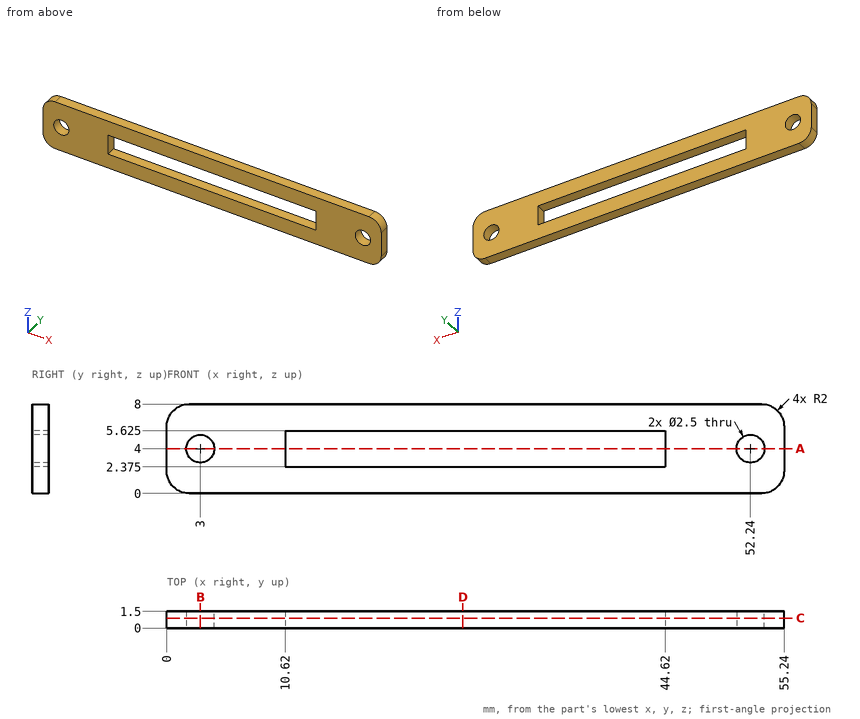
Here's the drawing with two shaded views (mm, measured from the low corner). I have some questions. Round coordinates to 2 decimals unless told otherwise and drop trailing zeros. Loops run counter-clockwise (first coordinate to the right, second up) from the corner with the lowest first, then second, coordinate; pieces in that order, holes last. Notation, with made-up numbers: (-26, 78) - (30, 78) arc R16 cw to (30, 108) - close; hole circle Ø1 at (85, 56). An arc over 180 degrees is marked (long way). Use CSV: the item, a comma, the result in double quotes.
Item 1: If we section it at A-A on z = 4: List the corners of the cut face in (x, y) for me.
Here are the results:
outline,"(0, 0) - (1.75, 0) - (1.75, 1.5) - (0, 1.5) - close; (4.25, 0) - (10.62, 0) - (10.62, 1.5) - (4.25, 1.5) - close; (44.62, 0) - (50.99, 0) - (50.99, 1.5) - (44.62, 1.5) - close; (53.49, 0) - (55.24, 0) - (55.24, 1.5) - (53.49, 1.5) - close"
Item 2: If we section it at C-C on y = 0.9: Count the separate pieces of the cut face and the enclosed holes in it, then the cut area to 3 significant figures.
Here are the results:
separate pieces,"1"
enclosed holes,"3"
area,"318 mm²"
Item 3: If we section it at B-B on x = 3: List the corners of the cut face in (y, z) for me.
Here are the results:
outline,"(0, 0) - (1.5, 0) - (1.5, 2.75) - (0, 2.75) - close; (0, 5.25) - (1.5, 5.25) - (1.5, 8) - (0, 8) - close"
Item 4: I need wall thicknesses on L1, parallel to X at y = 0.5, z = 4; L2, parallel to X at y = 0.45, z = 3.5 (1 decimal); L3, parallel to Z at x = 29, y = 0.4 (3 decimals). Which ranges of each line are inside material? Lowest first, please. Write a range as [from, to].
Here are the results:
L1,"x = [0, 1.75], [4.25, 10.62], [44.62, 50.99], [53.49, 55.24]"
L2,"x = [0, 1.9], [4.1, 10.6], [44.6, 51.1], [53.4, 55.2]"
L3,"z = [0, 2.375], [5.625, 8]"
Item 5: If we section it at D-D on x = 26.5: List the corners of the cut face in (y, z) for me (3 decimals).
Here are the results:
outline,"(0, 0) - (1.5, 0) - (1.5, 2.375) - (0, 2.375) - close; (0, 5.625) - (1.5, 5.625) - (1.5, 8) - (0, 8) - close"
